from build123d import *

# Parameters (mm, degrees)
SKETCH_1_W                      = 15
SKETCH_1_H                      = 15
EXTRUDE_1_DEPTH                 = 2
SKETCH_2_W                      = 3
SKETCH_2_H                      = 3
EXTRUDE_2_DEPTH                 = 1
EXTRUDE_3_DEPTH                 = 2
EXTRUDE_3_DEPTH_BACK            = 2
CUT_EXTRUDE_1_REACH             = 12.897
CUT_EXTRUDE_1_DIRECTION_2_REACH = 12.897
FILLET_1_R                      = 0.1
FILLET_2_R                      = 0.2


with BuildPart() as part:
    # 草图1 → 凸台-拉伸1 (new body)
    with BuildSketch(Plane.XY):
        Rectangle(SKETCH_1_W, SKETCH_1_H)
    extrude(amount=-EXTRUDE_1_DEPTH)

    # 草图2 → 凸台-拉伸2 (add)
    with BuildSketch(Plane.XY):
        Rectangle(SKETCH_2_W, SKETCH_2_H)
    extrude(amount=EXTRUDE_2_DEPTH)

    # 草图3 → 凸台-拉伸3 (add, two sides: drawn at the far end of the back side and taken through both)
    with BuildSketch(Plane(origin=(0, 0, 0), x_dir=(1, 0, 0), z_dir=(0, 1, 0)).offset(-EXTRUDE_3_DEPTH_BACK)):
        with BuildLine():
            Line((-1.95, -2.5), (1.95, -2.5))
            Line((1.95, -2.5), (1.95, -1.555590279))
            ThreePointArc((1.95, -1.555590279), (1.780042303, -1.088161527), (1.5, -0.677124344))
            Line((1.5, -0.677124344), (-1.5, -0.677124344))
            ThreePointArc((-1.5, -0.677124344), (-1.780042303, -1.088161527), (-1.95, -1.555590279))
            Line((-1.95, -1.555590279), (-1.95, -2.5))
        make_face()
    extrude(amount=EXTRUDE_3_DEPTH + EXTRUDE_3_DEPTH_BACK)

    # 草图4 → 切除-拉伸1 (cut, up to next)
    with BuildSketch(Plane(origin=(0, 0, 0), x_dir=(0, 0, -1), z_dir=(1, 0, 0)), mode=Mode.PRIVATE) as cut_extrude_1_sk1:
        with BuildLine():
            Line((-2.5, 1.95), (-1.555590279, 1.95))
            ThreePointArc((-1.555590279, 1.95), (-1.088161527, 1.780042303), (-0.677124344, 1.5))
            Line((-0.677124344, 1.5), (-0.677124344, 2))
            Line((-0.677124344, 2), (-2.5, 2))
            Line((-2.5, 2), (-2.5, 1.95))
        make_face()
    cut_extrude_1_tool1 = extrude(cut_extrude_1_sk1.sketch, amount=-CUT_EXTRUDE_1_REACH, mode=Mode.PRIVATE) & part.part
    # 草图4 → 切除-拉伸1 (cut, up to next)
    with BuildSketch(Plane(origin=(0, 0, 0), x_dir=(0, 0, -1), z_dir=(1, 0, 0)), mode=Mode.PRIVATE) as cut_extrude_1_sk2:
        with BuildLine():
            Line((-2.5, -2), (-0.677124344, -2))
            Line((-0.677124344, -2), (-0.677124344, -1.5))
            ThreePointArc((-0.677124344, -1.5), (-1.088161527, -1.780042303), (-1.555590279, -1.95))
            Line((-1.555590279, -1.95), (-2.5, -1.95))
            Line((-2.5, -1.95), (-2.5, -2))
        make_face()
    cut_extrude_1_tool2 = extrude(cut_extrude_1_sk2.sketch, amount=-CUT_EXTRUDE_1_REACH, mode=Mode.PRIVATE) & part.part
    add(cut_extrude_1_tool1.solids().sort_by_distance((0, 1.873038, 1.175075))[0], mode=Mode.SUBTRACT)
    add(cut_extrude_1_tool2.solids().sort_by_distance((0, -1.873038, 1.175075))[0], mode=Mode.SUBTRACT)

    # 草图4 → 切除-拉伸1 direction 2 (cut, up to next)
    with BuildSketch(Plane(origin=(0, 0, 0), x_dir=(0, 0, -1), z_dir=(1, 0, 0)), mode=Mode.PRIVATE) as cut_extrude_1_direction_2_sk1:
        with BuildLine():
            Line((-2.5, 1.95), (-1.555590279, 1.95))
            ThreePointArc((-1.555590279, 1.95), (-1.088161527, 1.780042303), (-0.677124344, 1.5))
            Line((-0.677124344, 1.5), (-0.677124344, 2))
            Line((-0.677124344, 2), (-2.5, 2))
            Line((-2.5, 2), (-2.5, 1.95))
        make_face()
    cut_extrude_1_direction_2_tool1 = extrude(cut_extrude_1_direction_2_sk1.sketch, amount=CUT_EXTRUDE_1_DIRECTION_2_REACH, mode=Mode.PRIVATE) & part.part
    # 草图4 → 切除-拉伸1 direction 2 (cut, up to next)
    with BuildSketch(Plane(origin=(0, 0, 0), x_dir=(0, 0, -1), z_dir=(1, 0, 0)), mode=Mode.PRIVATE) as cut_extrude_1_direction_2_sk2:
        with BuildLine():
            Line((-2.5, -2), (-0.677124344, -2))
            Line((-0.677124344, -2), (-0.677124344, -1.5))
            ThreePointArc((-0.677124344, -1.5), (-1.088161527, -1.780042303), (-1.555590279, -1.95))
            Line((-1.555590279, -1.95), (-2.5, -1.95))
            Line((-2.5, -1.95), (-2.5, -2))
        make_face()
    cut_extrude_1_direction_2_tool2 = extrude(cut_extrude_1_direction_2_sk2.sketch, amount=CUT_EXTRUDE_1_DIRECTION_2_REACH, mode=Mode.PRIVATE) & part.part
    add(cut_extrude_1_direction_2_tool1.solids().sort_by_distance((0, 1.873038, 1.175075))[0], mode=Mode.SUBTRACT)
    add(cut_extrude_1_direction_2_tool2.solids().sort_by_distance((0, -1.873038, 1.175075))[0], mode=Mode.SUBTRACT)

    # 圆角1
    fillet_1_edges = [part.edges().sort_by_distance(p)[0] for p in [
        (-1.95, 0, 2.5),
        (1.95, 0, 2.5),
        (0, -1.95, 2.5),
        (0, 1.95, 2.5),
    ]]
    fillet(fillet_1_edges, radius=FILLET_1_R)

    # 圆角2
    fillet_2_edges = [part.edges().sort_by_distance(p)[0] for p in [
        (7.5, 0, -2),
        (0, 7.5, -2),
        (-7.5, 0, -2),
        (0, 7.5, 0),
        (7.5, 0, 0),
        (0, -7.5, 0),
        (-7.5, 0, 0),
        (0, -7.5, -2),
        (-7.5, 7.5, -1),
        (7.5, 7.5, -1),
        (7.5, -7.5, -1),
        (-7.5, -7.5, -1),
    ]]
    fillet(fillet_2_edges, radius=FILLET_2_R)


solid = part.part
Build history of the part. All positions in model axes, mm. A direction names the side the tool comes from. Round coordinates to 2 decimals unless told otherwise and drop trailing zeros. Write each loop counter-clockwise with the first axis right and the second up, starting at its lowest first coordinate (ties: lowest second). Pieces come first, ordered by that corner, then holes. Notation, with made-up numbers: M 18,-26.5 L 61,-26.5 A17 ccw 61,-9.5 Z; hole C 73.25,54.25 d1. An arc over 180 degrees is marked long. Answer in a Markdown table with one row per item.
1. Saw through at C-C (z = 0.3). List the corners of the cut face in (x, y), and give its area (3 significant figures).
Geometry check:
| item | result |
|---|---|
| outline | M -1.5,-1.5 L 1.5,-1.5 L 1.5,1.5 L -1.5,1.5 Z |
| area | 9.00 mm2 |
2. Probe L1, parallel to Z at x = 2.75, y = -6; L2, parallel to Y at x = -0.5, z = 1.95; L3, parallel to Y at x = 1.25, z = 0.45. List the from-to ranges inside material, lowest first. Write a range as [from, to].
Geometry check:
| item | result |
|---|---|
| L1 | [-2, 0] |
| L2 | [-1.95, 1.95] |
| L3 | [-1.5, 1.5] |
3. Mould opens along Z. For faces 6 (the face through (1.78, -0.03, 1.09)), 7 (the face through (0, 1.95, 2)), 8 (the face through (0, 0, 2.5)) say: +Z half, -Z half, draft (parallel to the pull), parting line (faces both ways), or undercut.
Geometry check:
| item | result |
|---|---|
| face 6 | undercut |
| face 7 | draft |
| face 8 | +Z half |
4. Saw through at A-A (x = -5.5). List the corners of the cut face in (y, z).
Geometry check:
| item | result |
|---|---|
| outline | M -7.5,-1.8 A0.2 ccw -7.3,-2 L 7.3,-2 A0.2 ccw 7.5,-1.8 L 7.5,-0.2 A0.2 ccw 7.3,0 L -7.3,0 A0.2 ccw -7.5,-0.2 Z |
5. Which spindle directions (+Z, -Z, +X, -X, +Y, -Y) get a long thin tool onto all of the face, cutting with end or side? Do faces 1 (the face through (1.95, 0, 2)), 2 (the face through (0, -1.95, 2)), 3 (the face through (-0.027, -1.777, 1.082)), 4 (the face through (-1.95, 0, 2)), 5 (the face through (-1.777, -0.027, 1.082)). Say none if no direction does.
Geometry check:
| item | result |
|---|---|
| face 1 | +Z, +X, +Y, -Y |
| face 2 | +Z, +X, -X, -Y |
| face 3 | +X, -X, -Y |
| face 4 | +Z, -X, +Y, -Y |
| face 5 | -X, +Y, -Y |
6. Saw through at B-B (y = 0). List the corners of the cut face in (x, z).
Geometry check:
| item | result |
|---|---|
| outline | M -7.5,-1.8 A0.2 ccw -7.3,-2 L 7.3,-2 A0.2 ccw 7.5,-1.8 L 7.5,-0.2 A0.2 ccw 7.3,0 L 1.5,0 L 1.5,0.68 A2 ccw 1.95,1.56 L 1.95,2.4 A0.1 ccw 1.85,2.5 L -1.85,2.5 A0.1 ccw -1.95,2.4 L -1.95,1.56 A2 ccw -1.5,0.68 L -1.5,0 L -7.3,0 A0.2 ccw -7.5,-0.2 Z |
7. Flat gauge pins, fed straight in: P1, Ø0.5, axis at x = -0.5, z = 0.5, coming from the -Y side; P2, Ø0.7, axis at x = 0.5, z = 0.5, coming from the +Y side; P3, Ø1, axis at x = 2.5, z = 1, coming from the +Y side; P4, Ø0.5, axis at y = 0, z = 0, coming from the -X side. Where does each tip first touch, or does it go through?
Geometry check:
| item | result |
|---|---|
| P1 | y = -1.56 |
| P2 | y = 1.64 |
| P3 | through |
| P4 | x = -7.5 |
